Source: CAD feature listing. Evaluate the final solid. Frame: model axes, mm. Coordinates: 2 decimals unless noted, no trailing zeros. Write each loop counter-clockwise with the first axis right and the second up, starting at its lowest first coordinate (ties: lowest second). Pieces come first, ordered by that corner, then holes. Notation, with made-up numbers: (-20, 75) - (-11, 75) arc R31 ccw to (-11, 99) - close; hole circle Ø3 at (11, 11.5). An arc over 180 degrees is marked (long way). One line per question, with ' | ' between items.
from build123d import *

# Parameters (mm, degrees)
SKETCH1_R           = 1.4
BOSS_EXTRUDE1_DEPTH = 3


with BuildPart() as part:
    # Sketch1 → Boss-Extrude1 (new body)
    with BuildSketch(Plane(origin=(0, 0, 0), x_dir=(1, 0, 0), z_dir=(0, 1, 0))):
        with BuildLine():
            Line((0, -1.025278455), (0, -8.974734883))
            ThreePointArc((0, -8.974734883), (-0.301768682, -9.690607097), (-1.024946053, -9.974423682))
            Line((-1.024946053, -9.974423682), (-40.099818721, -8.999356383))
            ThreePointArc((-40.099818721, -8.999356383), (-44.000366387, -5.000286937), (-40.099870732, -1.001166763))
            Line((-40.099870732, -1.001166763), (-1.024959055, -0.025589981))
            ThreePointArc((-1.024959055, -0.025589981), (-0.301773337, -0.309401701), (0, -1.025278455))
        make_face()
        with Locations(Location((-40.000026017, -5.000260924, 0), (0, 0, 270))):
            Circle(SKETCH1_R, mode=Mode.SUBTRACT)
    extrude(amount=BOSS_EXTRUDE1_DEPTH)


solid = part.part
Item 1: Mould query, pull axis X, two halves, no side actions, for faces 1 (the face through (-22, 0, 5)), 2 (the face through (0, 1, 5)), 3 (the face through (-38.61, 1.48, 4.82)). Classes: pulls with the +X half, pulls with the -X half, needs draft (parallel to the pull), parting line crosses it, or undercut.
Check sheet entries:
face 1: needs draft | face 2: pulls with the +X half | face 3: undercut
Item 2: Cut plane C-C on x = -39.5. Return loops of the section in (y, z).
Check sheet entries:
outline: (0, 0.99) - (3, 0.99) - (3, 3.69) - (0, 3.69) - close; (0, 6.31) - (3, 6.31) - (3, 9.01) - (0, 9.01) - close
Item 3: Cut plane A-A on z = 5. Return loops of the section in (x, y), and give its area (3 significant figures).
Check sheet entries:
outline: (-44, 0) - (-41.4, 0) - (-41.4, 3) - (-44, 3) - close; (-38.6, 0) - (0, 0) - (0, 3) - (-38.6, 3) - close | area: 124 mm²
Item 4: Cut plane B-B on y = 1.75. Return loops of the section in (x, z), and give its area (3 significant figures).
Check sheet entries:
outline: (-40.1, 1) - (-1.02, 0.03) arc R1 ccw to (0, 1.03) - (0, 8.97) arc R1 ccw to (-1.02, 9.97) - (-40.1, 9) arc R4 ccw to start; hole circle Ø2.8 at (-40, 5) | area: 379 mm²
Item 5: Ray query, line 1 along Z through (x, y) = (-40, 2.5); line 2 along X through (y, z) = (0.95, 5.25); line 3 along X through (y, z) = (0.35, 4.5). Return the intervals inside material, ascending. Write a range as [from, to].
Check sheet entries:
line 1: [1, 3.6], [6.4, 9] | line 2: [-43.99, -41.38], [-38.62, 0] | line 3: [-43.97, -41.31], [-38.69, 0]
Item 6: Pin query (flat end, axial travel): pin 1 Ø4 at (x, z) = (-14, 7.5) entering from -Y. Return the tip coordinate at first contact, or that it passes through.
Check sheet entries:
pin 1: y = 0
Item 7: Cut plane D-D on x = -20. Return loops of the section in (y, z), and give its area (3 significant figures).
Check sheet entries:
outline: (0, 0.5) - (3, 0.5) - (3, 9.5) - (0, 9.5) - close | area: 27.0 mm²
